Here's how the part is built. I have some questions about the finished solid (model axes, mm). Coordinates: 2 decimals unless noted, no trailing zeros. Loops run counter-clockwise (first coordinate to the right, second up) from the corner with the lowest first, then second, coordinate; pieces in that order, holes last. Notation, with made-up numbers: (85, -37.5) - (113, -37.5) arc R8 ccw to (113, -25.5) - close; hole circle Ø10 at (-12.5, 50). An arc over 180 degrees is marked (long way). Use a Markdown table: item, result.
```python
from build123d import *

# Parameters (mm, degrees)
F0_W     = 50.8
F0_H     = 412.75
F0_W_2   = 23.167712307
F0_H_2   = 152.4
F0_H_3   = 69.3220067978
F0_H_4   = 387.4254058838
F0_H_5   = 235.4025873184
F0_H_6   = 25.4
F0_H_7   = 450.85
F1_DEPTH = 25.4


with BuildPart() as f1:
    # F0 (on Top) → F1 (new body)
    with BuildSketch(Plane.XY):
        with Locations((0, 206.375)):
            Rectangle(F0_W, F0_H)
        with Locations((-36.9838561535, 488.95)):
            Rectangle(F0_W_2, F0_H_2)
        with Locations((0, 488.95)):
            Rectangle(F0_W, F0_H_2)
        with Locations((36.9838561535, 488.95)):
            Rectangle(F0_W_2, F0_H_2)
        with Locations((-36.9838561535, 599.8110033989)):
            Rectangle(F0_W_2, F0_H_3)
        with Locations((36.9838561535, 599.8110033989)):
            Rectangle(F0_W_2, F0_H_3)
        Polygon((-48.567712307, 634.4720067978), (-25.4, 634.4720067978), (-25.4, 1021.8974126816), (-152.4, 1021.8974126816), (-152.4, 565.15), (-48.567712307, 565.15), align=None)
        with Locations((0, 828.1847097397)):
            Rectangle(F0_W, F0_H_4)
        Polygon((25.4, 1021.8974126816), (25.4, 634.4720067978), (48.567712307, 634.4720067978), (48.567712307, 565.15), (152.4, 565.15), (152.4, 1021.8974126816), align=None)
        with Locations((0, 1139.5987063408)):
            Rectangle(F0_W, F0_H_5)
        Polygon((-285.75, 1257.3), (-25.4, 1257.3), (-25.4, 1282.7), (-260.35, 1282.7), (-260.35, 1409.7), (-285.75, 1409.7), align=None)
        with Locations((0, 1270)):
            Rectangle(F0_W, F0_H_6)
        Polygon((25.4, 1282.7), (25.4, 1257.3), (285.75, 1257.3), (285.75, 1409.7), (260.35, 1409.7), (260.35, 1282.7), align=None)
        with Locations((0, 1508.125)):
            Rectangle(F0_W, F0_H_7)
        with Locations((0, 599.8110033989)):
            Rectangle(F0_W, F0_H_3)
    extrude(amount=F1_DEPTH)


solid = f1.part
```
Q1. Will these pins go through, and if not, where does the flat tip stop? P1, Ø7.5, axis at x = -118.5, z = 16, coming from the -Y side; P2, Ø12.5, axis at y = 1486.5, z = 9, coming from the +X side; P3, Ø3, axis at x = -195, z = 19.5, coming from the -Y side.
Check values:
| item | result |
|---|---|
| P1 | y = 565.15 |
| P2 | x = 25.4 |
| P3 | y = 1257.3 |
Q2. I want a section at D-D, the plane x = -212. Write out the boundary of the cut face in (y, z), then the cut area to 3 significant figures.
Check values:
| item | result |
|---|---|
| outline | (1257.3, 0) - (1282.7, 0) - (1282.7, 25.4) - (1257.3, 25.4) - close |
| area | 645 mm^2 |
Q3. I want a section at B-B, the plane z = 19. Write out the boundary of the cut face in (x, y), then the cut area to 3 significant figures.
Check values:
| item | result |
|---|---|
| outline | (-285.75, 1257.3) - (-25.4, 1257.3) - (-25.4, 1021.9) - (-152.4, 1021.9) - (-152.4, 565.15) - (-48.57, 565.15) - (-48.57, 412.75) - (-25.4, 412.75) - (-25.4, 0) - (25.4, 0) - (25.4, 412.75) - (48.57, 412.75) - (48.57, 565.15) - (152.4, 565.15) - (152.4, 1021.9) - (25.4, 1021.9) - (25.4, 1257.3) - (285.75, 1257.3) - (285.75, 1409.7) - (260.35, 1409.7) - (260.35, 1282.7) - (25.4, 1282.7) - (25.4, 1733.55) - (-25.4, 1733.55) - (-25.4, 1282.7) - (-260.35, 1282.7) - (-260.35, 1409.7) - (-285.75, 1409.7) - close |
| area | 231,000 mm^2 |
Q4. Please list where these lines run through material, in increasing order: L1, parallel to Y at x = -109, z = 18; L2, parallel to X at y = 243.5, z = 8.5; L3, parallel to Y at x = -253.5, z = 9. Write a range as from..to.
Check values:
| item | result |
|---|---|
| L1 | 565.15..1021.9, 1257.3..1282.7 |
| L2 | -25.4..25.4 |
| L3 | 1257.3..1282.7 |
Q5. I want a section at C-C, the plane y = 494. Write out the boundary of the cut face in (x, z), then the cut area to 3 significant figures.
Check values:
| item | result |
|---|---|
| outline | (-48.57, 0) - (48.57, 0) - (48.57, 25.4) - (-48.57, 25.4) - close |
| area | 2,470 mm^2 |
Q6. I want a section at A-A, the plane x = 131.5. Write out the boundary of the cut face in (y, z).
Check values:
| item | result |
|---|---|
| outline | (565.15, 0) - (1021.9, 0) - (1021.9, 25.4) - (565.15, 25.4) - close; (1257.3, 0) - (1282.7, 0) - (1282.7, 25.4) - (1257.3, 25.4) - close |
